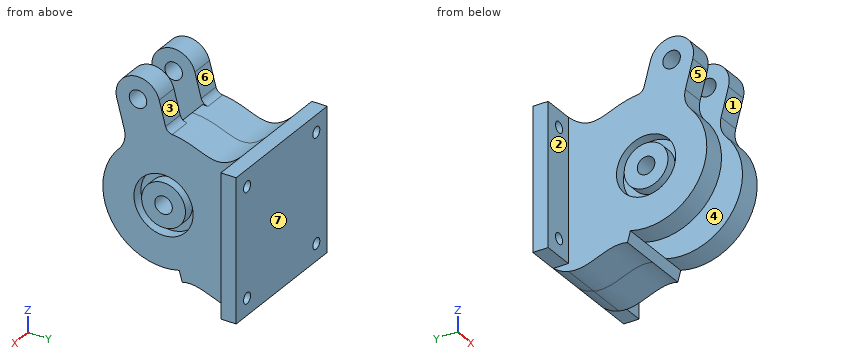
from build123d import *

# Parameters (mm, degrees)
SKETCH1_W                       = 65
SKETCH1_H                       = 65
SKETCH1_R                       = 2.5
BOSS_EXTRUDE1_DEPTH             = 7
BOSS_EXTRUDE2_START             = 7.5
SKETCH2_R                       = 4
BOSS_EXTRUDE2_DEPTH             = 10.5
BOSS_EXTRUDE3_REACH             = 80.065
BOSS_EXTRUDE3_DIRECTION_2_REACH = 80.065
BOSS_EXTRUDE7_START             = -18
BOSS_EXTRUDE7_DEPTH             = 36
SKETCH6_W                       = 15
SKETCH6_H                       = 30
CUT_EXTRUDE1_DEPTH              = 81.472268493
SKETCH8_R                       = 13.5
SKETCH8_R_2                     = 10
CUT_EXTRUDE3_DEPTH              = 5
CUT_EXTRUDE4_DEPTH              = 91.23260041
CUT_EXTRUDE4_DEPTH_BACK         = 91.23260041
SKETCH7_R                       = 4
FILLET16_R                      = 3.5
FILLET17_R                      = 3.5
FILLET19_R                      = 10


with BuildPart() as part:
    # Sketch1 → Boss-Extrude1 (new body)
    with BuildSketch(Plane(origin=(0, 0, 0), x_dir=(1, 0, 0), z_dir=(0, 1, 0))):
        Rectangle(SKETCH1_W, SKETCH1_H)
        with Locations(Location((-24.748737342, 24.748737342, 0), (0, 0, 270))):
            Circle(SKETCH1_R, mode=Mode.SUBTRACT)
        with Locations(Location((24.748737342, 24.748737342, 0), (0, 0, 270))):
            Circle(SKETCH1_R, mode=Mode.SUBTRACT)
        with Locations(Location((24.748737342, -24.748737342, 0), (0, 0, 270))):
            Circle(SKETCH1_R, mode=Mode.SUBTRACT)
        with Locations(Location((-24.748737342, -24.748737342, 0), (0, 0, 270))):
            Circle(SKETCH1_R, mode=Mode.SUBTRACT)
    extrude(amount=BOSS_EXTRUDE1_DEPTH)

    # Sketch2 → Boss-Extrude2 (add)
    with BuildSketch(Plane(origin=(0, 0, 0), x_dir=(0, 0, -1), z_dir=(1, 0, 0)).offset(BOSS_EXTRUDE2_START)):
        with BuildLine():
            Line((10, -9.568043047), (10, 1.517986249))
            Line((10, 1.517986249), (-10, 1.517986249))
            Line((-10, 1.517986249), (-10, -9.568043047))
            ThreePointArc((-10, -9.568043047), (0, -63.1), (10, -9.568043047))
        make_face()
        with Locations((0, -35.4)):
            Circle(SKETCH2_R, mode=Mode.SUBTRACT)
    boss_extrude2 = extrude(amount=BOSS_EXTRUDE2_DEPTH)

    # Mirror1: Boss-Extrude2 across plane
    add(boss_extrude2.mirror(Plane(origin=(0, 0, 0), x_dir=(0, 0, 1), z_dir=(1, 0, 0))))

    # Boss-Extrude3: up to this face of the body (flat: up to its plane)
    boss_extrude3_end = Plane(part.part.faces().sort_by_distance((18, -62.260311367, 0))[0])
    # Sketch3 → Boss-Extrude3 (add, up to the picked face)
    with BuildSketch(Plane(origin=(0, 0, 0), x_dir=(0, 0, -1), z_dir=(1, 0, 0)), mode=Mode.PRIVATE) as boss_extrude3_sk1:
        with BuildLine():
            Line((32.5, 0), (10, 0))
            Line((10, 0), (10, -4.266577445))
            Line((10, -4.266577445), (10, -9.568043047))
            ThreePointArc((10, -9.568043047), (20.611340647, -16.894253954), (26.756145388, -28.230712451))
            Line((26.756145388, -28.230712451), (31.61497925, -26.928791841))
            add(Edge.make_bspline(
                [(31.61497925, -26.928791841), (29.055948241, -17.442715383), (38.347474054, -9.80951762), (36, 0)],
                knots=[0, 0, 0, 0, 1, 1, 1, 1], degree=3))
            add(Edge.make_bspline(
                [(36, 0), (35.140208775, 3.592856394), (34.071491306, 4.753858958), (32.5, 7)],
                knots=[0, 0, 0, 0, 1, 1, 1, 1], degree=3))
            Line((32.5, 7), (32.5, 0))
        make_face()
    boss_extrude3_tool1 = split(extrude(boss_extrude3_sk1.sketch, amount=BOSS_EXTRUDE3_REACH, mode=Mode.PRIVATE), bisect_by=boss_extrude3_end, keep=Keep.BOTH, mode=Mode.PRIVATE)
    # Sketch3 → Boss-Extrude3 (add, up to the picked face)
    with BuildSketch(Plane(origin=(0, 0, 0), x_dir=(0, 0, -1), z_dir=(1, 0, 0)), mode=Mode.PRIVATE) as boss_extrude3_sk2:
        with BuildLine():
            Line((-32.5, 0), (-10, 0))
            Line((-10, 0), (-10, -9.568043047))
            ThreePointArc((-10, -9.568043047), (-24.698665766, -22.859429463), (-26.756145388, -42.569287549))
            Line((-26.756145388, -42.569287549), (-31.58577452, -43.863382775))
            add(Edge.make_bspline(
                [(-31.58577452, -43.863382775), (-37.603765688, -19.008690412), (-18.117487997, -15.033656142), (-32.5, 0)],
                knots=[0, 0, 0, 0, 1, 1, 1, 1], degree=3))
        make_face()
    boss_extrude3_tool2 = split(extrude(boss_extrude3_sk2.sketch, amount=BOSS_EXTRUDE3_REACH, mode=Mode.PRIVATE), bisect_by=boss_extrude3_end, keep=Keep.BOTH, mode=Mode.PRIVATE)
    add(boss_extrude3_tool1.solids().sort_by(Axis((0, -9.525708, -24.617363), (1, 0, 0)))[0])
    add(boss_extrude3_tool2.solids().sort_by(Axis((0, -14.994615, 23.210716), (1, 0, 0)))[0])

    # Boss-Extrude3 direction 2: up to this face of the body (flat: up to its plane)
    boss_extrude3_direction_2_end = Plane(part.part.faces().sort_by_distance((-18, -62.260311367, 0))[0])
    # Sketch3 → Boss-Extrude3 direction 2 (add, up to the picked face)
    with BuildSketch(Plane(origin=(0, 0, 0), x_dir=(0, 0, -1), z_dir=(1, 0, 0)), mode=Mode.PRIVATE) as boss_extrude3_direction_2_sk1:
        with BuildLine():
            Line((32.5, 0), (10, 0))
            Line((10, 0), (10, -4.266577445))
            Line((10, -4.266577445), (10, -9.568043047))
            ThreePointArc((10, -9.568043047), (20.611340647, -16.894253954), (26.756145388, -28.230712451))
            Line((26.756145388, -28.230712451), (31.61497925, -26.928791841))
            add(Edge.make_bspline(
                [(31.61497925, -26.928791841), (29.055948241, -17.442715383), (38.347474054, -9.80951762), (36, 0)],
                knots=[0, 0, 0, 0, 1, 1, 1, 1], degree=3))
            add(Edge.make_bspline(
                [(36, 0), (35.140208775, 3.592856394), (34.071491306, 4.753858958), (32.5, 7)],
                knots=[0, 0, 0, 0, 1, 1, 1, 1], degree=3))
            Line((32.5, 7), (32.5, 0))
        make_face()
    boss_extrude3_direction_2_tool1 = split(extrude(boss_extrude3_direction_2_sk1.sketch, amount=-BOSS_EXTRUDE3_DIRECTION_2_REACH, mode=Mode.PRIVATE), bisect_by=boss_extrude3_direction_2_end, keep=Keep.BOTH, mode=Mode.PRIVATE)
    # Sketch3 → Boss-Extrude3 direction 2 (add, up to the picked face)
    with BuildSketch(Plane(origin=(0, 0, 0), x_dir=(0, 0, -1), z_dir=(1, 0, 0)), mode=Mode.PRIVATE) as boss_extrude3_direction_2_sk2:
        with BuildLine():
            Line((-32.5, 0), (-10, 0))
            Line((-10, 0), (-10, -9.568043047))
            ThreePointArc((-10, -9.568043047), (-24.698665766, -22.859429463), (-26.756145388, -42.569287549))
            Line((-26.756145388, -42.569287549), (-31.58577452, -43.863382775))
            add(Edge.make_bspline(
                [(-31.58577452, -43.863382775), (-37.603765688, -19.008690412), (-18.117487997, -15.033656142), (-32.5, 0)],
                knots=[0, 0, 0, 0, 1, 1, 1, 1], degree=3))
        make_face()
    boss_extrude3_direction_2_tool2 = split(extrude(boss_extrude3_direction_2_sk2.sketch, amount=-BOSS_EXTRUDE3_DIRECTION_2_REACH, mode=Mode.PRIVATE), bisect_by=boss_extrude3_direction_2_end, keep=Keep.BOTH, mode=Mode.PRIVATE)
    add(boss_extrude3_direction_2_tool1.solids().sort_by(Axis((0, -9.525708, -24.617363), (-1, 0, 0)))[0])
    add(boss_extrude3_direction_2_tool2.solids().sort_by(Axis((0, -14.994615, 23.210716), (-1, 0, 0)))[0])

    # Sketch4 → Boss-Extrude7 (add)
    with BuildSketch(Plane(origin=(0, 0, 0), x_dir=(0, 0, -1), z_dir=(1, 0, 0)).offset(BOSS_EXTRUDE7_START)):
        with BuildLine():
            Line((-27.539944815, -32.426544169), (-33.139527425, -33.926947807))
            Line((-33.139527425, -33.926947807), (-55.714110897, -39.975789218))
            Line((-55.714110897, -39.975789218), (-50.537729995, -59.294305744))
            Line((-50.537729995, -59.294305744), (-22.363563913, -51.745060694))
            ThreePointArc((-22.363563913, -51.745060694), (-26.756145388, -42.569287549), (-27.539944815, -32.426544169))
        make_face()
    extrude(amount=BOSS_EXTRUDE7_DEPTH)

    # Sketch6 → Cut-Extrude1 (cut, through all)
    with BuildSketch(Plane(origin=(0, -23.369391384, -6.261809549), x_dir=(1, 0, 0), z_dir=(0, 0.9659258262890686, 0.2588190451025195))):
        with Locations((0, -49.162194197)):
            Rectangle(SKETCH6_W, SKETCH6_H)
    extrude(amount=-CUT_EXTRUDE1_DEPTH, mode=Mode.SUBTRACT)

    # Sketch8 → Cut-Extrude3 (cut)
    with BuildSketch(Plane(origin=(18, 0, 0), x_dir=(0, 0, -1), z_dir=(1, 0, 0))):
        with Locations((0, -35.4)):
            Circle(SKETCH8_R)
        with Locations((0, -35.4)):
            Circle(SKETCH8_R_2, mode=Mode.SUBTRACT)
    cut_extrude3 = extrude(amount=-CUT_EXTRUDE3_DEPTH, mode=Mode.SUBTRACT)

    # Mirror2: Cut-Extrude3 across plane
    add(cut_extrude3.mirror(Plane(origin=(0, 0, 0), x_dir=(0, 0, 1), z_dir=(1, 0, 0))), mode=Mode.SUBTRACT)

    # Sketch7 → Cut-Extrude4 (cut, two sides: drawn at the far end of the back side and taken through both)
    with BuildSketch(Plane(origin=(0, 0, 0), x_dir=(0, 0, -1), z_dir=(1, 0, 0)).offset(-CUT_EXTRUDE4_DEPTH_BACK)):
        with Locations(Location((-43.466662183, -47.04685703, 0), (0, 0, 180))):
            Circle(SKETCH7_R)
        with BuildLine():
            Line((-40.878471732, -56.706115293), (-40.166415946, -59.363543662))
            Line((-40.166415946, -59.363543662), (-53.107989986, -62.831227975))
            Line((-53.107989986, -62.831227975), (-59.564338385, -38.735807717))
            Line((-59.564338385, -38.735807717), (-46.622764346, -35.268123405))
            Line((-46.622764346, -35.268123405), (-46.054852634, -37.387598767))
            ThreePointArc((-46.054852634, -37.387598767), (-53.125920446, -49.635047481), (-40.878471732, -56.706115293))
        make_face()
    extrude(amount=CUT_EXTRUDE4_DEPTH + CUT_EXTRUDE4_DEPTH_BACK, mode=Mode.SUBTRACT)

    # Fillet16
    # the kernel refuses this fillet: 3.5 mm, written as the material it adds along each edge
    with BuildSketch(Plane(origin=(18, -33.827938234, 32.770018668), x_dir=(0, -0.25881904510252074, 0.9659258262890684), z_dir=(-1, 0, 0))) as fillet16_piece_1_section:
        with BuildLine():
            CenterArc((2.528363882, 3.5), FILLET16_R, 200.393732709, 69.606267291)
            Line((-0.752256512, 2.280356677), (-0.81786892, 2.255963811))
            ThreePointArc((-0.81786892, 2.255963811), (-0.421453854, 1.125231743), (-0.06723899, -0.019465823))
            Line((-0.06723899, -0.019465823), (0, -0.07))
            Line((0, -0.07), (2.528363882, -0.07))
            Line((2.528363882, -0.07), (2.528363882, 0))
        make_face()
    fillet16_piece_1 = extrude(amount=10.5, mode=Mode.PRIVATE)
    fillet16_piece_1 = split(fillet16_piece_1, bisect_by=Plane(origin=(12.75, -33.904495307, 33.055733556), z_dir=(0, 0.9659258262890686, 0.2588190451025195)), keep=Keep.TOP, mode=Mode.PRIVATE)
    add(fillet16_piece_1)

    # Fillet17
    # the kernel refuses this fillet: 3.5 mm, written as the material it adds along each edge
    with BuildSketch(Plane(origin=(-18, -33.827938234, 32.770018668), x_dir=(0, -0.25881904510252074, 0.9659258262890684), z_dir=(1, 0, 0))) as fillet17_piece_1_section:
        with BuildLine():
            CenterArc((2.528363882, -3.5), FILLET17_R, 90, 69.606267291)
            Line((-0.752256512, -2.280356677), (-0.81786892, -2.255963811))
            ThreePointArc((-0.81786892, -2.255963811), (-0.421453854, -1.125231743), (-0.06723899, 0.019465823))
            Line((-0.06723899, 0.019465823), (0, 0.07))
            Line((0, 0.07), (2.528363882, 0.07))
            Line((2.528363882, 0.07), (2.528363882, 0))
        make_face()
    fillet17_piece_1 = extrude(amount=10.5, mode=Mode.PRIVATE)
    fillet17_piece_1 = split(fillet17_piece_1, bisect_by=Plane(origin=(-12.75, -33.904495307, 33.055733556), z_dir=(0, 0.9659258262890686, 0.2588190451025195)), keep=Keep.TOP, mode=Mode.PRIVATE)
    add(fillet17_piece_1)

    # Fillet19
    fillet19_edges = [part.edges().sort_by_distance(p)[0] for p in [
        (12.75, -51.745060694, 22.363563913),
        (-12.75, -51.745060694, 22.363563913),
    ]]
    fillet(fillet19_edges, radius=FILLET19_R)


solid = part.part
Model file for the job. Use its own axes, mm. Face numbers are marked on the shaded views. A direction names the side the tool comes from. Give positions to 0.01 mm unless a question says otherwise; leave off trailing zeros. Order: outer loops, then holes, each group sorted by start corner. A loop starts at its lowest first (then second) coordinate and runs counter-clockwise, first axis right, second up. Notation, with made-up numbers: (-40, 32) - (-12, 32) arc R16 cw to (-12, 59) - close; hole circle Ø6 at (24, -29.5). An arc over 180 degrees is marked (long way). One line per item, written item: value.
Item 1: Pin check, flat tips, straight feed: pin 1 Ø21.5 at (y, z) = (-35.4, 0) entering from +X; pin 2 Ø5 at (y, z) = (-35.4, 0) entering from +X; pin 3 Ø5 at (x, y) = (2.5, -5) entering from -Z; pin 4 Ø4 at (x, z) = (-2.5, -6.5) entering from -Y. Stop position of each tip, or through.
Response values:
pin 1: x = 18
pin 2: through
pin 3: z = -36.38
pin 4: y = 0
Item 2: Slice it at D-D (z = 24.5). List the corners of the cut face in (x, y).
Response values:
outline: (-32.5, 0) - (-27.24, 0) - (-27.24, 7) - (-32.5, 7) - close; (-22.26, 0) - (-18, 0) - (-18, -53.06) - (-7.5, -53.06) - (-7.5, -22.48) - (7.5, -22.48) - (7.5, -53.06) - (18, -53.06) - (18, 0) - (22.26, 0) - (22.26, 7) - (-22.26, 7) - close; (27.24, 0) - (32.5, 0) - (32.5, 7) - (27.24, 7) - close
Item 3: Slice it at B-B (z = 0). Give the number of separate pieces and of enclosed holes in the cut face, then the cut area to 3 significant figures.
Response values:
separate pieces: 3
enclosed holes: 0
area: 1,540 mm2
Item 4: Wall check: line 1 (Y direction, x = -13.95, z = 0); line 2 (X direction, y = -41.5, z = 40); line 3 (Y direction, x = 0, z = -4). Give the ranges that are in metal, low to high.
Response values:
line 1: -63.1 to -48.9, -45.4 to -39.4, -31.4 to -25.4, -21.9 to 7
line 2: -18 to -7.5, 7.5 to 18
line 3: 0 to 7
Item 5: Tool access for the marked faces 1, 2, 3 and 4: list every direction of +Z, -Z, +X, -X, +Y, -Y with a clear straight run to the whole face (end or side of a thin tool).
Response values:
face 1: +X, -X, -Y
face 2: +Z, -Z, -X, -Y
face 3: +Z, +X, -X, +Y
face 4: -Y
Item 6: Slice it at C-C (z = -15). List the corners of the cut face in (x, y).
Response values:
outline: (-32.5, 0) - (-18, 0) - (-18, -58.69) - (-7.5, -58.69) - (-7.5, -12.11) - (7.5, -12.11) - (7.5, -58.69) - (18, -58.69) - (18, 0) - (32.5, 0) - (32.5, 7) - (-32.5, 7) - close
Item 7: Slice it at A-A (z = 42). List the corners of the cut face in (x, y), then the cut area to 3 significant figures.
Response values:
outline: (-18, -56.94) - (-7.5, -56.94) - (-7.5, -50.77) - (-18, -50.77) - close; (-18, -43.33) - (-7.5, -43.33) - (-7.5, -36.3) - (-18, -36.3) - close; (7.5, -56.94) - (18, -56.94) - (18, -50.77) - (7.5, -50.77) - close; (7.5, -43.33) - (18, -43.33) - (18, -36.3) - (7.5, -36.3) - close
area: 277 mm2
Item 8: Two-plate mould, pull along Z, no slides. Class the marked faces 5, 6 and 7: released by +Z, released by -Z, zero draft, split by the parting line, or undercut.
Response values:
face 5: undercut
face 6: released by +Z
face 7: zero draft
